Part model, mm, in its own coordinate system. Face numbers are marked on the shaded views. A direction names the side the tool comes from. Coordinates: 2 decimals unless noted, no trailing zeros. Loops run counter-clockwise (first coordinate to the right, second up) from the corner with the lowest first, then second, coordinate; pieces in that order, holes last. Notation, with made-up numbers: (-1, -2.5) - (47, -2.5) arc R10 cw to (47, 9.5) - close; hole circle Ø5 at (-4, 22). An arc over 180 degrees is marked (long way). Use a Markdown table: item, result. Add a question column.
1) Pull direction Z, two halves, no side cores. Call the marked faces 1, 2 and 3: +Z half, -Z half, draft (parallel to the pull), parting line (faces both ways), or undercut.
2) Probe probe 1 along Z at (x, y) = (-10.7, 24.1); probe 2 along Z at (x, y) = (-10, 23); probe 3 along Y at (x, z) = (-1.5, 25). List the from-to ranges inside material, lowest first. Write a range as [from, to].
3) Band-saw the part on A-A (x = 0). Give the cut face in (y, z).
4) Band-saw the part on D-D (x = -37.5). Give the cut face in (y, z), plus the area to 3 significant figures.
5) Drop flat-ended pins along their axis: P1, Ø4.5, axis at x = 5, y = -4, coming from the -Z side; P2, Ø1.7, axis at x = 2, y = -2.5, coming from the +Z side; P3, Ø4.5, axis at y = -2.5, z = 34.5, coming from the -X side. Give the stop position or say it passes through.
6) Band-saw the part on B-B (z = -27.5). Give the cut face in (x, y).
7) Tool access for the marked faces 4, 5, 6 and 7: list every direction of +Z, -Z, +X, -X, +Y, -Y with a clear straight run to the whole face (end or side of a thin tool).
8) Band-saw the part on C-C (y = 7). Give the cut face in (x, z).
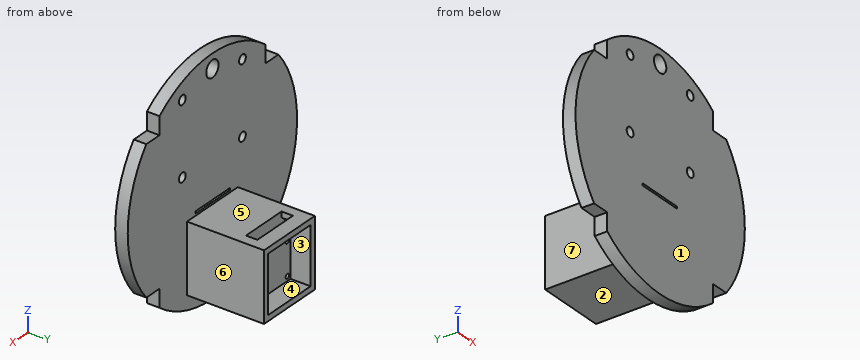
Autodesk Fusion 360 part; units mm, degrees
sketch "Sketch1" plane through (0, 0, 0) normal (0, 1, 0) x (1, 0, 0)
  arc A0 (31.75, 39.6557) -> (-31.75, 39.6557) centre (0, 0) ccw
  arc A1 (39.6557, -31.75) -> (39.6557, 31.75) centre (0, 0) ccw
  arc A2 (-39.6557, 31.75) -> (-39.6557, -31.75) centre (0, 0) ccw
  arc A3 (-31.75, -39.6557) -> (31.75, -39.6557) centre (0, 0) ccw
  line L0 (-31.75, -39.6557) -> (-31.75, -31.75)
  line L1 (-31.75, 31.75) -> (-31.75, 39.6557)
  line L2 (39.6557, 31.75) -> (31.75, 31.75)
  line L3 (-31.75, 31.75) -> (-39.6557, 31.75)
  line L4 (31.75, 39.6557) -> (31.75, 31.75)
  line L5 (31.75, -31.75) -> (31.75, -39.6557)
  line L6 (-39.6557, -31.75) -> (-31.75, -31.75)
  line L7 (31.75, -31.75) -> (39.6557, -31.75)
  dimension "d1" = 101.6
sketch "Sketch2" plane through (0, 0, 0) normal (0, 1, 0) x (1, 0, 0)
  circle A0 centre (-18.034, -7.874) radius 2.032
  circle A1 centre (18.034, -7.874) radius 2.032
  circle A2 centre (-18.034, -39.878) radius 2.032
  circle A3 centre (18.034, -39.878) radius 2.032
  dimension "d9" = 36.068
  dimension "d11" = 32.004
  dimension "d12" = 36.068
  dimension "d13" = 4.064
  dimension "d14" = 4.064
  dimension "d15" = 4.064
  dimension "d16" = 4.064
extrude "Extrude1" add sketch "Sketch1" against normal blind 5.588
sketch "Sketch4" plane through (0, 0, 0) normal (0, 1, 0) x (1, 0, 0)
  circle A0 centre (18.034, -39.878) radius 2.032
  line L0 (12.7, 39.6369) -> (12.7, 14.2369)
  line L1 (15.24, 11.6969) -> (-15.24, 11.6969)
  line L2 (-12.7, 14.2369) -> (-12.7, 39.6369)
  line L3 (15.24, 42.1769) -> (15.24, 11.6969)
  line L4 (12.7, 14.2369) -> (-12.7, 14.2369)
  circle A1 centre (18.034, -7.874) radius 2.032
  line L5 (-15.24, 42.1769) -> (15.24, 42.1769)
  circle A2 centre (-18.034, -39.878) radius 2.032
  line L6 (-12.7, 39.6369) -> (12.7, 39.6369)
  circle A3 centre (-18.034, -7.874) radius 2.032
  line L7 (-15.24, 11.6969) -> (-15.24, 42.1769)
  dimension "d29" = 36.068
  dimension "d30" = 32.004
  dimension "d31" = 36.068
  dimension "d32" = 4.064
  dimension "d33" = 4.064
  dimension "d34" = 4.064
  dimension "d35" = 4.064
extrude "Extrude2" cut sketch "Sketch2" against normal blind 22
extrude "Extrude3" add sketch "Sketch4" along normal blind 34.29 contours L1 L3 L5 L7
extrude "Extrude4" add 1 faces at (-4.2333, 0, -31.1702) along direction (0, 1, 0) blind 25.4
sketch "Sketch5" plane through (0, 25.4, 0) normal (0, 1, 0) x (-1, 0, 0)
  line L0 (12.7, -14.2369) -> (-12.7, -14.2369)
  line L1 (-12.7, -14.2369) -> (-12.7, -39.6369)
  line L2 (-12.7, -39.6369) -> (12.7, -39.6369)
  line L3 (12.7, -39.6369) -> (12.7, -14.2369)
  line L4 (12.7, -14.2369) -> (-12.7, -14.2369)
  line L5 (-12.7, -14.2369) -> (-12.7, -19.8249)
  line L6 (-12.7, -19.8249) -> (12.7, -19.8249)
  line L7 (12.7, -19.8249) -> (12.7, -14.2369)
  dimension "d42" = 5.588
extrude "Extrude5" cut sketch "Sketch5" against normal blind 2.54 contours L0 L1 L3 L4 L5 L6 L7
sketch "Sketch6" plane through (0, 0, -14.2369) normal (0, 0, -1) x (-1, 0, 0)
  line L0 (12.7, 22.86) -> (12.7, 34.29)
  line L1 (12.7, 34.29) -> (-12.7, 34.29)
  line L2 (-12.7, 34.29) -> (-12.7, 22.86)
  line L3 (-12.7, 22.86) -> (12.7, 22.86)
  line L4 (-10.668, 27.94) -> (10.668, 27.94)
  line L5 (10.668, 27.94) -> (10.668, 22.86)
  line L6 (10.668, 22.86) -> (-10.668, 22.86)
  line L7 (-10.668, 22.86) -> (-10.668, 27.94)
extrude "Extrude6" cut sketch "Sketch6" against normal blind 17 contours L3 L4 L5 L6 L7
sketch "Sketch7" plane through (0, 0, -11.6969) normal (0, 0, 1) x (1, 0, 0)
  line L0 (-10.668, 22.86) -> (-10.668, 27.94)
  line L1 (-10.668, 27.94) -> (10.668, 27.94)
  line L2 (10.668, 27.94) -> (10.668, 22.86)
  line L3 (10.668, 22.86) -> (-10.668, 22.86)
  line L4 (-15.24, 0) -> (15.24, 0)
  line L5 (15.24, 0) -> (15.24, 34.29)
  line L6 (15.24, 34.29) -> (-15.24, 34.29)
  line L7 (-15.24, 34.29) -> (-15.24, 0)
sketch "Sketch8" plane through (0, 25.4, 0) normal (0, 1, 0) x (-1, 0, 0)
  line L0 (12.7, -19.8249) -> (-12.7, -19.8249)
  line L1 (-12.7, -19.8249) -> (-12.7, -39.6369)
  line L2 (-12.7, -39.6369) -> (12.7, -39.6369)
  line L3 (12.7, -39.6369) -> (12.7, -19.8249)
  circle A0 centre (10.7, -37.6369) radius 1
  circle A1 centre (-10.7, -37.6369) radius 1
  circle A2 centre (10.7, -23.1369) radius 1
  circle A3 centre (-10.7, -23.1369) radius 1
  dimension "d53" = 2
  dimension "d54" = 2
  dimension "d56" = 2
  dimension "d57" = 2
extrude "Extrude7" cut sketch "Sketch8" against normal blind 4 contours A0 | A1 | A2 | A3
sketch "Sketch9" plane through (0, 0, 0) normal (0, 1, 0) x (-1, 0, 0)
  arc A0 (31.75, 39.6557) -> (-31.75, 39.6557) centre (0, 0) ccw
  line L0 (-31.75, 39.6557) -> (-31.75, 31.75)
  line L1 (-31.75, 31.75) -> (-39.6557, 31.75)
  arc A1 (-39.6557, 31.75) -> (-39.6557, -31.75) centre (0, 0) ccw
  line L2 (-39.6557, -31.75) -> (-31.75, -31.75)
  line L3 (-31.75, -31.75) -> (-31.75, -39.6557)
  arc A2 (-31.75, -39.6557) -> (31.75, -39.6557) centre (0, 0) ccw
  line L4 (31.75, -39.6557) -> (31.75, -31.75)
  line L5 (31.75, -31.75) -> (39.6557, -31.75)
  arc A3 (39.6557, -31.75) -> (39.6557, 31.75) centre (0, 0) ccw
  line L6 (39.6557, 31.75) -> (31.75, 31.75)
  line L7 (31.75, 31.75) -> (31.75, 39.6557)
  circle A4 centre (18.034, 7.874) radius 2.032
  circle A5 centre (18.034, 39.878) radius 2.032
  circle A6 centre (-18.034, 7.874) radius 2.032
  circle A7 centre (-18.034, 39.878) radius 2.032
  line L8 (15.24, -11.6969) -> (15.24, -42.1769)
  line L9 (15.24, -42.1769) -> (-15.24, -42.1769)
  line L10 (-15.24, -42.1769) -> (-15.24, -11.6969)
  line L11 (-15.24, -11.6969) -> (15.24, -11.6969)
  circle A8 centre (0, 44.3767) radius 3.6975
extrude "Extrude8" cut sketch "Sketch9" against normal blind 17 contours A8
sketch "Sketch10" plane through (0, 0, 0) normal (0, 1, 0) x (1, 0, 0)
  line L0 (-15.24, 11.6969) -> (15.24, 11.6969)
  line L1 (15.24, 10.2652) -> (14.8192, 10.2652)
  line L2 (10.668, 14.2369) -> (10.668, 11.6969)
  line L3 (-10.668, 9.8177) -> (10.2472, 9.8177)
  line L4 (10.2472, 9.8177) -> (10.2472, 10.7473)
  line L5 (10.2472, 10.7473) -> (-10.668, 10.7473)
  line L6 (-10.668, 10.7473) -> (-10.668, 9.8177)
  point P0 (-15.24, 11.6969)
extrude "Extrude9" cut sketch "Sketch10" against normal blind 14
Answer block:
| question | item | result |
|---|---|---|
| 1 | face 1 | draft |
| 1 | face 2 | -Z half |
| 1 | face 3 | undercut |
| 2 | probe 1 | [-42.18, -38.64], [-36.64, -24.14], [-22.14, -19.82], [-14.24, -11.7] |
| 2 | probe 2 | [-42.18, -38.35], [-36.92, -23.85], [-22.42, -19.82] |
| 2 | probe 3 | [-5.59, 0] |
| 3 | outline | (-5.59, -50.8) - (0, -50.8) - (0, -42.18) - (34.29, -42.18) - (34.29, -39.64) - (25.4, -39.64) - (25.4, -19.82) - (22.86, -19.82) - (22.86, -11.7) - (0, -11.7) - (0, -10.75) - (-5.59, -10.75) - close; (-5.59, -9.82) - (0, -9.82) - (0, 40.68) - (-5.59, 40.68) - close; (-5.59, 48.07) - (0, 48.07) - (0, 50.8) - (-5.59, 50.8) - close; (27.94, -14.24) - (34.29, -14.24) - (34.29, -11.7) - (27.94, -11.7) - close |
| 4 | outline | (-5.59, -31.75) - (0, -31.75) - (0, 31.75) - (-5.59, 31.75) - close |
| 4 | area | 355 mm2 |
| 5 | P1 | z = -50.73 |
| 5 | P2 | z = 50.79 |
| 5 | P3 | x = -31.75 |
| 6 | outline | (-42.71, -5.59) - (42.71, -5.59) - (42.71, 0) - (15.24, 0) - (15.24, 34.29) - (12.7, 34.29) - (12.7, 25.4) - (-12.7, 25.4) - (-12.7, 34.29) - (-15.24, 34.29) - (-15.24, 0) - (-42.71, 0) - close |
| 7 | face 4 | +Y |
| 7 | face 5 | +Z, +X, -X, +Y |
| 7 | face 6 | +Z, -Z, +X, +Y |
| 7 | face 7 | +Z, -Z, -X, +Y |
| 8 | outline | (-15.24, -42.18) - (15.24, -42.18) - (15.24, -11.7) - (-15.24, -11.7) - close |
